from build123d import *

# Parameters (mm, degrees)
F0_R     = 80
F1_DEPTH = 600
F2_R     = 25
F3_DEPTH = 100


with BuildPart() as f1:
    # F0 (on Front) → F1 (new body, symmetric)
    with BuildSketch(Plane.XZ):
        Circle(F0_R)
    extrude(amount=F1_DEPTH, both=True)

    # F2 (on face) → F3 (join)
    with BuildSketch(Plane.XZ.offset(600)):
        Circle(F2_R)
    extrude(amount=F3_DEPTH)

    # F4: F1 across plane


with BuildPart() as f1_1:
    add(f1.part)
    add(f1.part.mirror(Plane.XZ))


solid = f1_1.part
Verification items for the finished model (mm, model axes). A direction names the side the tool comes from. Coordinates: 2 decimals unless noted, no trailing zeros. Order: outer loops, then holes, each group sorted by start corner. A loop starts at its lowest first (then second) coordinate and runs counter-clockwise, first axis right, second up. Notation, with made-up numbers: M 44,-40 L 87,-40 A24 ccw 87,-24 Z; hole C -21,3 d2. An arc over 180 degrees is marked long. Return JSON: item names as keys, results as strings.
1) Access from +Z, -Z, +X, -X, +Y, -Y to the whole of each face (thin tool, end or side, straight path). Record for faces 1 (the flat face through (17, 600, 19)), 2 (the cylindrical face through (-17.34, -8.4, -78.1)), 3 (the flat face through (17, -600, 19)).
Answer list:
{"face 1": "+Y", "face 2": "+Y, -Y", "face 3": "-Y"}
2) Cross-section at C-C, the plane y = -531. Record the boundary of the cut face in (x, z).
Answer list:
{"outline": "C 0,0 d160"}
3) Thickness scan on L1, parallel to Y at x = -19, z = 40; L2, parallel to X at y = 0.5, z = 3.5; L3, parallel to Z at x = 63, y = 597. Record the ranges inside material, lowest first. Write a range as [from, to].
Answer list:
{"L1": "[-600, 600]", "L2": "[-79.92, 79.92]", "L3": "[-49.31, 49.31]"}
4) Cross-section at B-B, the plane x = 0. Record the boundary of the cut face in (y, z), and give its area (3 significant figures).
Answer list:
{"outline": "M -700,-25 L -600,-25 L -600,-80 L 600,-80 L 600,-25 L 700,-25 L 700,25 L 600,25 L 600,80 L -600,80 L -600,25 L -700,25 Z", "area": "202,000 mm2"}
5) Cross-section at A-A, the plane z = 0. Record the boundary of the cut face in (x, y), and give its area (3 significant figures).
Answer list:
{"outline": "M -80,-600 L -25,-600 L -25,-700 L 25,-700 L 25,-600 L 80,-600 L 80,600 L 25,600 L 25,700 L -25,700 L -25,600 L -80,600 Z", "area": "202,000 mm2"}
6) Gauge pin test, flat ends, axial feed: pin 1 (1 mm diameter, centred on x = 30, z = -60.5, fed in from -Y); pin 2 (10 mm diameter, centred on x = -47, y = -388, fed in from -Z); pin 3 (2 mm diameter, centred on x = 22, y = 126.5, fed in from -Z). Record the tip position at first contact, or that the pin passes through.
Answer list:
{"pin 1": "y = -600", "pin 2": "z = -68.09", "pin 3": "z = -77.19"}
